```python
from build123d import *

# Parameters (mm, degrees)
SKETCH1_R           = 17.5
BOSS_EXTRUDE2_DEPTH = 40
SKETCH1_3_R         = 2.5
BOSS_EXTRUDE3_DEPTH = 19
SKETCH1_4_R         = 5.5
BOSS_EXTRUDE4_DEPTH = 42
SKETCH1_5_R         = 3
BOSS_EXTRUDE5_DEPTH = 70
SKETCH1_6_R         = 7.5
BOSS_EXTRUDE6_DEPTH = 46.5
FILLET1_R           = 1
FILLET2_R           = 3


with BuildPart() as part:
    # Sketch1 → Boss-Extrude2 (new body)
    with BuildSketch(Plane.XY):
        Circle(SKETCH1_R)
    extrude(amount=BOSS_EXTRUDE2_DEPTH)

    # Sketch1_3 → Boss-Extrude3 (add)
    with BuildSketch(Plane.XY):
        Circle(SKETCH1_3_R)
    extrude(amount=-BOSS_EXTRUDE3_DEPTH)

    # Sketch1_4 → Boss-Extrude4 (add)
    with BuildSketch(Plane.XY):
        with Locations(Location((0, 0, 0), (0, 0, 180))):
            Circle(SKETCH1_4_R)
    extrude(amount=BOSS_EXTRUDE4_DEPTH)

    # Sketch1_5 → Boss-Extrude5 (add)
    with BuildSketch(Plane.XY):
        Circle(SKETCH1_5_R)
    extrude(amount=BOSS_EXTRUDE5_DEPTH)

    # Sketch1_6 → Boss-Extrude6 (add)
    with BuildSketch(Plane.XY):
        with Locations(Location((0, 0, 0), (0, 0, 180))):
            Circle(SKETCH1_6_R)
    extrude(amount=BOSS_EXTRUDE6_DEPTH)

    # Fillet1
    fillet1_edges = [part.edges().sort_by_distance(p)[0] for p in [
        (-17.5, 0, 40),
    ]]
    fillet(fillet1_edges, radius=FILLET1_R)

    # Fillet2
    fillet2_edges = [part.edges().sort_by_distance(p)[0] for p in [
        (-17.5, 0, 0),
    ]]
    fillet(fillet2_edges, radius=FILLET2_R)


solid = part.part
```
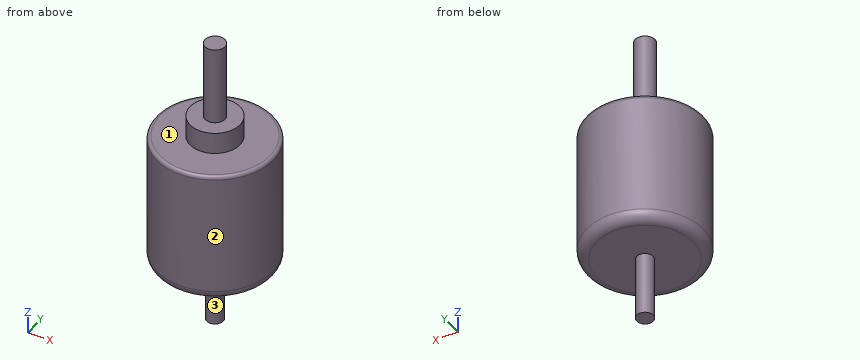
Geometry: final body of the model. Coordinates: model frame, mm. Face numbers are marked on the shaded views. A direction names the side the tool comes from. Coordinates: 2 decimals unless noted, no trailing zeros. Order: outer loops, then holes, each group sorted by start corner. A loop starts at its lowest first (then second) coordinate and runs counter-clockwise, first axis right, second up. Notation, with made-up numbers: (-19, 78.5) -> (6, 78.5) arc R27 ccw to (6, 96.5) -> close; hole circle Ø2 at (81.25, 37). An arc over 180 degrees is marked (long way). Write each question's results on one line, items separated by ' | '. Start each with the question number.
1) Cut plane A-A, the plane y = 0. Output: boundary loops of the cut face in (x, z).
2) Cut plane C-C, the plane z = 60.5. Output: boundary loops of the cut face in (x, y).
3) Set-up query: the marked faces 1, 2 and 3. Return all of +Z, -Z, +X, -X, +Y, -Y with unobstructed straight access to the full face (end or side cutting, diameter ignored); none if empty.
4) Material intervals for line 1 along Z through (x, y) = (9, 0.5); line 2 along Z through (x, y) = (-1, 4); line 3 along Y through (x, z) = (-0.5, 29), sorted ascending.
5) Cut plane D-D, the plane z = -11. Output: boundary loops of the cut face in (x, y).
6) First-contact query: pin 1 (6 mm diameter, centred on x = 4, y = 11.5, fed in from +Z); pin 2 (4 mm diameter, centred on y = 4, z = -3.5, fed in from -X); pin 3 (6 mm diameter, centred on y = -6.5, z = 18, fed in from -X). Flat tips, straight axial feed; report the tip coordinate or a pass-through.
Checks:
1) outline: (-17.5, 3) arc R3 ccw to (-14.5, 0) -> (-2.5, 0) -> (-2.5, -19) -> (2.5, -19) -> (2.5, 0) -> (14.5, 0) arc R3 ccw to (17.5, 3) -> (17.5, 39) arc R1 ccw to (16.5, 40) -> (7.5, 40) -> (7.5, 46.5) -> (3, 46.5) -> (3, 70) -> (-3, 70) -> (-3, 46.5) -> (-7.5, 46.5) -> (-7.5, 40) -> (-16.5, 40) arc R1 ccw to (-17.5, 39) -> close
2) outline: circle Ø6 at (0, 0)
3) face 1: +Z | face 2: +Z, -Z | face 3: -Z
4) line 1: 0 to 40 | line 2: 0 to 46.5 | line 3: -17.49 to 17.49
5) outline: circle Ø5 at (0, 0)
6) pin 1: z = 40 | pin 2: x = -1.5 | pin 3: x = -17.15
